Geometry: final body of the model. Coordinates: model frame, mm. A direction names the side the tool comes from. Coordinates: 2 decimals unless noted, no trailing zeros. Loops run counter-clockwise (first coordinate to the right, second up) from the corner with the lowest first, then second, coordinate; pieces in that order, holes last. Notation, with made-up numbers: (11, -21.5) -> (49, -21.5) arc R28 ccw to (49, 3.5) -> close; hole circle Ø11 at (59, 3). An arc over 180 degrees is marked (long way). One line per item, written item: value. Start each with the question number.
Item 1: Contact query for flat-ended pins moving along their axis: pin 1 Ø2 at (x, z) = (0, -15.5) entering from -Y; pin 2 Ø2 at (y, z) = (-3, 17.5) entering from -X; pin 3 Ø4 at (y, z) = (2.5, 12.5) entering from +X; pin 4 Ø1.4 at (y, z) = (0.5, 23.5) entering from -X. Output: stop coordinate, or through.
Item 2: Mould query, pull axis Y, two halves, no side actions, for faces 4 (the flat face through (0, 0, -27.5)), 5 (the cylindrical face through (5, 0, -11)), 6 (the flat face through (2.028, 3.448, 22.887)). Classes: +Y half, -Y half, draft (parallel to the pull), parting line (faces both ways), or undercut.
Item 3: Ray query, probe 1 along Y at (x, z) = (6.25, 24); probe 2 along Z at (x, y) = (5.25, 5.25); probe 3 along X at (y, z) = (1.25, 11). Return the intervals inside material, ascending. Write a range as from..to.
Item 4: Set-up query: faces 1 (the flat face through (4, 0, 23)), 2 (the cylindrical face through (1.009, -7.684, 18.5)), 3 (the flat face through (5, 2, 27.5)). Return all of +Z, -Z, +X, -X, +Y, -Y with unobstructed straight access to the full face (end or side cutting, diameter ignored); none if empty.
Item 5: Section query B-B on z = 15. Return loops of the section in (x, y).
Item 6: Section query A-A on z = -2. Return loops of the section in (x, y).
from build123d import *

# Parameters (mm, degrees)
CUT_EXTRUDE1_DEPTH = 9


with BuildPart() as part:
    # Sketch2 → Revolve1 (revolve)
    with BuildSketch(Plane(origin=(0, 0, 0), x_dir=(0, 0, -1), z_dir=(1, 0, 0)), mode=Mode.PRIVATE) as revolve1_sk:
        with BuildLine():
            Line((-27.5, 0), (-27.5, 7.448223305))
            ThreePointArc((-27.5, 7.448223305), (-27.490484942, 7.496058734), (-27.463388348, 7.536611652))
            Line((-27.463388348, 7.536611652), (-27.036611652, 7.963388348))
            ThreePointArc((-27.036611652, 7.963388348), (-26.996058734, 7.990484942), (-26.948223305, 8))
            Line((-26.948223305, 8), (-19.676776695, 8))
            ThreePointArc((-19.676776695, 8), (-19.628941266, 7.990484942), (-19.588388348, 7.963388348))
            Line((-19.588388348, 7.963388348), (-19.411611652, 7.786611652))
            ThreePointArc((-19.411611652, 7.786611652), (-19.371058734, 7.759515058), (-19.323223305, 7.75))
            Line((-19.323223305, 7.75), (-17.7, 7.75))
            ThreePointArc((-17.7, 7.75), (-17.558578644, 7.691421356), (-17.5, 7.55))
            Line((-17.5, 7.55), (-17.5, 5.662379763))
            ThreePointArc((-17.5, 5.662379763), (-17.353553391, 5.308826373), (-17, 5.162379763))
            Line((-17, 5.162379763), (-6.001952451, 5.162379763))
            ThreePointArc((-6.001952451, 5.162379763), (-5.879431025, 5.156360672), (-5.758089548, 5.138361364))
            Line((-5.758089548, 5.138361364), (-5.183248648, 5.024018399))
            ThreePointArc((-5.183248648, 5.024018399), (-5.061907171, 5.006019092), (-4.939385746, 5))
            Line((-4.939385746, 5), (26.525721421, 5))
            Line((26.525721421, 5), (27.5, 4.025721421))
            Line((27.5, 4.025721421), (27.5, 0))
            Line((27.5, 0), (-27.5, 0))
        make_face()
    revolve(revolve1_sk.sketch.rotate(Axis((0, 0, -27.5), (0, 0, 1)), 90), axis=Axis((0, 0, -27.5), (0, 0, 1)))

    # Sketch3 → Cut-Extrude1 (cut)
    with BuildSketch(Plane.XY.offset(27.5)):
        Polygon((4, -2.309401077), (4, 2.309401077), (0, 4.618802154), (-4, 2.309401077), (-4, -2.309401077), (0, -4.618802154), align=None)
    extrude(amount=-CUT_EXTRUDE1_DEPTH, mode=Mode.SUBTRACT)

    # Cut-Extrude2 cone 1 section (through the dimple's axis) → Cut-Extrude2 (revolve, cut)
    with BuildSketch(Plane(origin=(0, 0, 27.5), x_dir=(0, -1, 0), z_dir=(1, 0, 0))):
        Polygon((0, 0), (4.965212315, 0), (0, 4.965212315), align=None)
    revolve(axis=Axis((0, 0, 27.5), (0, 0, -1)), mode=Mode.SUBTRACT)


solid = part.part
Reply:
1. pin 1: stops at y = -5
1. pin 2: stops at x = -7.48
1. pin 3: stops at x = 5.14
1. pin 4: stops at x = -8
2. face 4: draft
2. face 5: parting line
2. face 6: undercut
3. probe 1: y = -4.99..4.99
3. probe 2: z = 17.5..27.5
3. probe 3: x = -5.01..5.01
4. face 1: +Z
4. face 2: -Z
4. face 3: +Z, +X, -X, +Y, -Y
5. outline: circle Ø10.32 at (0, 0)
6. outline: circle Ø10 at (0, 0)
